from build123d import *

# Parameters (mm, degrees)
F0_R     = 14
F1_DEPTH = 3.5
F2_DEPTH = 10
F3_START = 8
F3_DEPTH = 2
F4_R     = 1


with BuildPart() as f1:
    # F0 (on Front) → F1 (new body)
    with BuildSketch(Plane.XZ):
        with BuildLine():
            ThreePointArc((2.6195479008, -15.7841049412), (12.2047688715, -10.3461885153), (16, 0))
            ThreePointArc((16, 0), (-10.3461885153, 12.2047688715), (-2.6195479008, -15.7841049412))
            ThreePointArc((-2.6195479008, -15.7841049412), (0, -14.9760404944), (2.6195479008, -15.7841049412))
        make_face()
        Circle(F0_R, mode=Mode.SUBTRACT)
    extrude(amount=-F1_DEPTH)

    # F0 (on Front) → F2 (join)
    with BuildSketch(Plane.XZ):
        with BuildLine():
            ThreePointArc((2.6195479008, -15.7841049412), (0, -14.9760404944), (-2.6195479008, -15.7841049412))
            ThreePointArc((-2.6195479008, -15.7841049412), (0, -16), (2.6195479008, -15.7841049412))
        make_face()
        with BuildLine():
            ThreePointArc((2.6195479008, -15.7841049412), (12.2047688715, -10.3461885153), (16, 0))
            ThreePointArc((16, 0), (-10.3461885153, 12.2047688715), (-2.6195479008, -15.7841049412))
            ThreePointArc((-2.6195479008, -15.7841049412), (0, -14.9760404944), (2.6195479008, -15.7841049412))
        make_face()
        Circle(F0_R, mode=Mode.SUBTRACT)
    extrude(amount=F2_DEPTH)

    # F0 (on Front) → F3 (join)
    with BuildSketch(Plane.XZ.offset(F3_START)):
        Circle(F0_R)
    extrude(amount=F3_DEPTH)

    # F4
    f4_edges = [f1.edges().sort_by_distance(p)[0] for p in [
        (-2.619548, -10, 15.784105),
        (-14, 3.5, 0),
    ]]
    fillet(f4_edges, radius=F4_R)


solid = f1.part
Check sheet for the modelled part. Datum: model origin and axes. Units: mm. A direction names the side the tool comes from. Give positions to 0.01 mm unless a question says otherwise; leave off trailing zeros. Write each loop counter-clockwise with the first axis right and the second up, starting at its lowest first coordinate (ties: lowest second). Pieces come first, ordered by that corner, then holes. Notation, with made-up numbers: (28.25, 44) -> (57.25, 44) arc R12 cw to (57.25, 63) -> close; hole circle Ø11 at (22.5, -15.75). An arc over 180 degrees is marked (long way). One line per item, written item: value. Start each with the question number.
Item 1: Material ranges on probe 1 along X at (y, z) = (0, 0); probe 2 along Y at (x, z) = (0, -5.5), recorded low to high. Write a range as from..to.
Item 2: Tool access check on faces 1 (the flat face through (0, 0, -15.5)), 2 (the flat face through (0, -8, 0)), 3 (the flat face through (11, 3.5, 11)). Record the directions out of +Z, -Z, +X, -X, +Y, -Y that give a thin tool (end or side, any length) a straight path to the whole face; none if there is none.
Item 3: Gauge pin test, flat ends, axial feed: pin 1 (1.5 mm diameter, centred on x = -2, y = 2, fed in from -Z); pin 2 (4 mm diameter, centred on x = -5.5, y = -8, fed in from -Z); pin 3 (0.5 mm diameter, centred on x = 1, z = -15.5, fed in from +Y). Record the tip position at first contact, or that the pin passes through.
Item 4: Section check A-A on y = 0.5. Record the cut outline in (x, z).
Results list:
1. probe 1: -16..-14, 14..16
1. probe 2: -10..-8
2. face 1: -Z, +Y
2. face 2: +Y
2. face 3: +Z, -Z, +X, -X, +Y
3. pin 1: z = -15.78
3. pin 2: z = -15.61
3. pin 3: y = 0
4. outline: (-2.62, -15.78) arc R4.65 cw to (2.62, -15.78) arc R16 ccw (long way) to start; hole circle Ø28 at (0, 0)
